Source: CAD feature listing. Evaluate the final solid. Frame: model axes, mm. A direction names the side the tool comes from. Give positions to 0.01 mm unless a question says otherwise; leave off trailing zeros. Order: outer loops, then holes, each group sorted by start corner. A loop starts at its lowest first (then second) coordinate and runs counter-clockwise, first axis right, second up. Notation, with made-up numbers: M 58,-35 L 65,-35 A17 cw 65,-5 Z; hole C -38,77 d8. An arc over 180 degrees is marked long. Return JSON: item names as keys, results as strings.
from build123d import *

# Parameters (mm, degrees)
F0_W          = 90
F0_H          = 90
F1_DEPTH      = 70
F2_W          = 86
F2_H          = 86
F3_DEPTH      = 65
F4_R          = 4.5
F5_DEPTH      = 70
F6_W          = 30
F6_H          = 35
F7_DEPTH      = 2
F8_R          = 1.25
F9_DEPTH      = 15
F10_R         = 4
F10_R_2       = 1.25
F11_DEPTH     = 13
F12_T1_DEPTH  = 2
F12_T3_DEPTH  = 65
F12_T8_DEPTH  = 73.9443680268
F12_T13_DEPTH = 65


# Not quite as in the source:
# - a fillet or chamfer that OpenCascade refuses, or shapes differently, is made with other operations: its cross-section is extruded or revolved along the edge and cut away or added
# - a feature of the source that left no trace in its solid (it failed there, or was rolled back) is left out


with BuildPart() as f1:
    # F0 (on Top) → F1 (new body)
    with BuildSketch(Plane.XY):
        with Locations((45, 45)):
            Rectangle(F0_W, F0_H)
    extrude(amount=F1_DEPTH)

    # F2 (on face) → F3 (cut)
    with BuildSketch(Plane.XY.offset(70)):
        with Locations((45, 45)):
            Rectangle(F2_W, F2_H)
    extrude(amount=-F3_DEPTH, mode=Mode.SUBTRACT)

    # F4 (on Top) → F5 (join)
    with BuildSketch(Plane.XY):
        with Locations((2, 88)):
            Circle(F4_R)
        with Locations((88, 88)):
            Circle(F4_R)
        with Locations((2, 2)):
            Circle(F4_R)
        with Locations((88, 2)):
            Circle(F4_R)
    extrude(amount=F5_DEPTH)

    # F6 (on Front) → F7 (cut, through all)
    with BuildSketch(Plane.XZ):
        with Locations((25, 52.5)):
            Rectangle(F6_W, F6_H)
    extrude(amount=-F7_DEPTH, mode=Mode.SUBTRACT)

    # F8 (on face) → F9 (cut)
    with BuildSketch(Plane.XY.offset(70)):
        with Locations((2, 88)):
            Circle(F8_R)
        with Locations((88, 88)):
            Circle(F8_R)
        with Locations((2, 2)):
            Circle(F8_R)
        with Locations((88, 2)):
            Circle(F8_R)
    extrude(amount=-F9_DEPTH, mode=Mode.SUBTRACT)

    # F10 (on face) → F11 (join)
    with BuildSketch(Plane.XY.offset(5)):
        with Locations((19, 73)):
            Circle(F10_R)
        with Locations((19, 73)):
            Circle(F10_R_2, mode=Mode.SUBTRACT)
        with Locations((83, 73)):
            Circle(F10_R)
        with Locations((83, 73)):
            Circle(F10_R_2, mode=Mode.SUBTRACT)
        with Locations((83, 14)):
            Circle(F10_R)
        with Locations((83, 14)):
            Circle(F10_R_2, mode=Mode.SUBTRACT)
        with Locations((19, 14)):
            Circle(F10_R)
        with Locations((19, 14)):
            Circle(F10_R_2, mode=Mode.SUBTRACT)
    extrude(amount=F11_DEPTH)

    # F12: fillet of radius 5 on 10 edges, made by hand

    # F12_s2 → F12_t1 (join)
    with BuildSketch(Plane.XZ.offset(-2)):
        with BuildLine():
            ThreePointArc((40, 40), (38.5355339059, 36.4644660941), (35, 35))
            Line((35, 35), (40, 35))
            Line((40, 35), (40, 40))
        make_face()
        with BuildLine():
            ThreePointArc((15, 35), (11.4644660941, 36.4644660941), (10, 40))
            Line((10, 40), (10, 35))
            Line((10, 35), (15, 35))
        make_face()
    extrude(amount=F12_T1_DEPTH)

    # F12_s4 → F12_t3 (join)
    with BuildSketch(Plane.XY.offset(5)):
        with BuildLine():
            ThreePointArc((79.9222527893, 2), (82.3555741063, 2.6320545598), (84.1736986897, 4.3684210526))
            ThreePointArc((84.1736986897, 4.3684210526), (83.6717003398, 3.2311872529), (83.5, 2))
            Line((83.5, 2), (79.9222527893, 2))
        make_face()
        with BuildLine():
            ThreePointArc((85.6315789474, 5.8263013103), (87.3679454402, 7.6444258937), (88, 10.0777472107))
            Line((88, 10.0777472107), (88, 6.5))
            ThreePointArc((88, 6.5), (86.7688127471, 6.3282996602), (85.6315789474, 5.8263013103))
        make_face()
        with BuildLine():
            ThreePointArc((4.3684210526, 5.8263013103), (2.6320545598, 7.6444258937), (2, 10.0777472107))
            Line((2, 10.0777472107), (2, 6.5))
            ThreePointArc((2, 6.5), (3.2311872529, 6.3282996602), (4.3684210526, 5.8263013103))
        make_face()
        with BuildLine():
            ThreePointArc((88, 79.9222527893), (87.3679454402, 82.3555741063), (85.6315789474, 84.1736986897))
            ThreePointArc((85.6315789474, 84.1736986897), (86.7688127471, 83.6717003398), (88, 83.5))
            Line((88, 83.5), (88, 79.9222527893))
        make_face()
        with BuildLine():
            ThreePointArc((2, 79.9222527893), (2.6320545598, 82.3555741063), (4.3684210526, 84.1736986897))
            ThreePointArc((4.3684210526, 84.1736986897), (3.2311872529, 83.6717003398), (2, 83.5))
            Line((2, 83.5), (2, 79.9222527893))
        make_face()
        with BuildLine():
            ThreePointArc((84.1736986897, 85.6315789474), (82.3555741063, 87.3679454402), (79.9222527893, 88))
            Line((79.9222527893, 88), (83.5, 88))
            ThreePointArc((83.5, 88), (83.6717003398, 86.7688127471), (84.1736986897, 85.6315789474))
        make_face()
        with BuildLine():
            ThreePointArc((5.8263013103, 85.6315789474), (7.6444258937, 87.3679454402), (10.0777472107, 88))
            Line((10.0777472107, 88), (6.5, 88))
            ThreePointArc((6.5, 88), (6.3282996602, 86.7688127471), (5.8263013103, 85.6315789474))
        make_face()
    extrude(amount=F12_T3_DEPTH)


with BuildPart() as f12_tool6:
    # F12_s7 → F12_t8 (new body)
    with BuildSketch(Plane.XY.offset(5)):
        with BuildLine():
            ThreePointArc((10.0777472107, 2), (7.6444258937, 2.6320545598), (5.8263013103, 4.3684210526))
            ThreePointArc((5.8263013103, 4.3684210526), (6.3282996602, 3.2311872529), (6.5, 2))
            Line((6.5, 2), (10.0777472107, 2))
        make_face()
    extrude(amount=F12_T8_DEPTH)

    split(bisect_by=Plane.XY.offset(35), keep=Keep.BOTTOM)


with BuildPart() as f1_1:
    add(f1.part)

    # F12_t5: union F12_tool6
    add(f12_tool6.part)


with BuildPart() as f12_tool11:
    # F12_s12 → F12_t13 (new body)
    with BuildSketch(Plane.XY.offset(5)):
        with BuildLine():
            ThreePointArc((10.0777472107, 2), (7.6444258937, 2.6320545598), (5.8263013103, 4.3684210526))
            ThreePointArc((5.8263013103, 4.3684210526), (6.3282996602, 3.2311872529), (6.5, 2))
            Line((6.5, 2), (10.0777472107, 2))
        make_face()
    extrude(amount=F12_T13_DEPTH)

    split(bisect_by=Plane.YZ.offset(10), keep=Keep.BOTTOM)


with BuildPart() as f1_2:
    add(f1_1.part)

    # F12_t10: union F12_tool11
    add(f12_tool11.part)


solid = f1_2.part
1. Section query A-A (z = 62.5). State how many separate pieces and enclosed holes the cut face has, then the cut area to 3 significant figures.
Evaluation:
{"separate pieces": "1", "enclosed holes": "4", "area": "808 mm^2"}
2. First-contact query: pin 1 (3 mm diameter, centred on x = 88, y = 2, fed in from +Z); pin 2 (2.5 mm diameter, centred on x = 81.5, y = 73.5, fed in from +Z); pin 3 (12 mm diameter, centred on x = 63, y = 81.5, fed in from +Z); pin 4 (0.8 mm diameter, centred on x = 88, y = 88, fed in from +Z). Flat tips, straight axial feed; report the tip coordinate or a pass-through.
Evaluation:
{"pin 1": "stops at z = 70", "pin 2": "stops at z = 18", "pin 3": "stops at z = 5", "pin 4": "stops at z = 55"}
3. Ray query, probe 1 along Y at (x, z) = (19, 12); probe 2 along X at (y, z) = (42, 54.5); probe 3 along Y at (x, z) = (83, 13.5). Return the intervals inside material, ascending.
Evaluation:
{"probe 1": "y = 0 to 2, 10 to 12.75, 15.25 to 18, 69 to 71.75, 74.25 to 77, 88 to 90", "probe 2": "x = 0 to 2, 88 to 90", "probe 3": "y = 0 to 3.06, 10 to 12.75, 15.25 to 18, 69 to 71.75, 74.25 to 77, 86.94 to 90"}
4. Section query D-D (y = 14). Return loops of the section in (x, z).
Evaluation:
{"outline": "M 0,0 L 90,0 L 90,70 L 88,70 L 88,5 L 87,5 L 87,18 L 84.25,18 L 84.25,5 L 81.75,5 L 81.75,18 L 79,18 L 79,5 L 23,5 L 23,18 L 20.25,18 L 20.25,5 L 17.75,5 L 17.75,18 L 15,18 L 15,5 L 2,5 L 2,70 L 0,70 Z"}
5. Section query B-B (x = 45.5). Return loops of the section in (y, z).
Evaluation:
{"outline": "M 0,0 L 90,0 L 90,70 L 88,70 L 88,5 L 2,5 L 2,70 L 0,70 Z"}
6. Draft query along X for faces 4 (the face through (19.672, 15.054, 11.409)), 5 (the face through (90, 44, 35)). Return one class per face: pulls with the +X half, pulls with the -X half, needs draft (parallel to the pull), parting line crosses it, or undercut.
Evaluation:
{"face 4": "undercut", "face 5": "pulls with the +X half"}
7. Set-up query: faces 1 (the face through (1.84, 89.24, 62.6)), 2 (the face through (44, 90, 35)), 3 (the face through (44, 0, 35)). Return all of +Z, -Z, +X, -X, +Y, -Y with unobstructed straight access to the full face (end or side cutting, diameter ignored); none if empty.
Evaluation:
{"face 1": "+Z", "face 2": "+Z, -Z, +Y", "face 3": "+Z, -Z, -Y"}
